```python
from build123d import *

# Parameters (mm, degrees)
SKETCH001_W       = 0.6
SKETCH001_H       = 18.5
PAD001_DEPTH      = 3
PAD002_DEPTH      = 9
PAD002_DEPTH_BACK = 3
FILLET_R          = 1
FILLET001_R       = 2


with BuildPart() as part:
    # Sketch001 → Pad001 (new body)
    with BuildSketch(Plane.YZ):
        Polygon((-13, 10.5), (-13, -10.5), (0, -10.5), (0, -7.5), (-7, -7.5), (-7, 7.5), (0, 7.5), (0, 21.5), (-2.5, 21.5), (-5, 10.5), align=None)
        with Locations((-11, 0)):
            Rectangle(SKETCH001_W, SKETCH001_H, mode=Mode.SUBTRACT)
    extrude(amount=PAD001_DEPTH)

    # Sketch002 (on Face16 of Pad001) → Pad002 (join, two sides)
    with BuildSketch(Plane.YZ.offset(3)) as pad002_sk:
        with BuildLine():
            ThreePointArc((-2.457456, 26.343228), (-2.661032, 23.237253), (0, 21.622499))
            Line((0, 21.622499), (0, 20.622499))
            ThreePointArc((-3.276608, 26.916805), (-3.548043, 22.775505), (0, 20.622499))
            Line((-2.457456, 26.343228), (-3.276608, 26.916805))
        make_face()
    extrude(amount=PAD002_DEPTH)
    extrude(pad002_sk.sketch, amount=-PAD002_DEPTH_BACK)

    # Mirrored: part across XZ


with BuildPart() as part_1:
    add(part.part)
    add(part.part.mirror(Plane.XZ))

    # Fillet
    fillet_edges = [part_1.edges().sort_by_distance(p)[0] for p in [
        (1.5, 13, 10.5),
        (1.5, 13, -10.5),
        (1.5, -13, -10.5),
        (1.5, -13, 10.5),
    ]]
    fillet(fillet_edges, radius=FILLET_R)

    # Fillet001
    fillet001_edges = [part_1.edges().sort_by_distance(p)[0] for p in [
        (1.5, -5, 10.5),
        (1.5, 5, 10.5),
    ]]
    fillet(fillet001_edges, radius=FILLET001_R)


solid = part_1.part
```
Could you check a few things on this model? Use its own coordinates, in mm. A direction names the side the tool comes from. Coordinates: 2 decimals unless noted, no trailing zeros. Write each loop counter-clockwise with the first axis right and the second up, starting at its lowest first coordinate (ties: lowest second). Pieces come first, ordered by that corner, then holes. Notation, with made-up numbers: (64, 32.25) -> (123, 32.25) arc R22 cw to (123, 54.25) -> close; hole circle Ø3 at (-20, -35.5). An arc over 180 degrees is marked (long way). Write item = value, one per line. Start each with the question number.
(1) I need wall thicknesses on line 1 (Y direction, x = 2, z = 6); line 2 (Z direction, x = 1.5, y = 6.75); line 3 (Z direction, x = 2, y = -11.25). Which ranges of each line are inside material? Lowest first, please. Write a range as [from, to].
(2) I want a section at C-C (y = -5.5). Please give me the cut outline in (x, z), plus the area to 3 significant figures.
(3) Which directions (+Z, -Z, +X, -X, +Y, -Y) give clear straight access to the entire face, cutting with the end or side of a thin tool? Please do faces 1 (the face through (1.48, 3.56, 16.84)), 2 (the face through (1, -10.7, 0)), 3 (the face through (1, -9, 10.5)), 4 (the face through (6.084, -2.861, 26.626)).
(4) I want a section at B-B (z = 0.5). Please give me the cut outline in (x, y).
(5) I want a section at D-D (x = 8.5). Please give me the cut outline in (y, z), plus the area to 3 significant figures.
(6) Will these pins go through, and if not, where does the flat tip stop? pin 1 (1.5 mm diameter, centred on y = -4.5, z = 8.5, fed in from -X); pin 2 (6 mm diameter, centred on x = 4.5, y = 8, fed in from +Z); pin 3 (1.5 mm diameter, centred on x = 2, y = -10, fed in from +Z); pin 4 (2 mm diameter, centred on x = 5, y = -4, fed in from -Z).
(7) I want a section at A-A (x = 2.25). Give the number of separate pieces and of enclosed holes in the cut face, plus the area to 3 significant figures.
(8) We'd pull the mould along Z, two halves only. Please class faces 5 (the face through (6.084, 2.861, 26.626)), 6 (the face through (12, 0, 21)), 7 (the face through (1, 11.3, 0)): released by +Z, released by -Z, zero draft, split by the parting line, or undercut.
Result set:
q1.line_1 = [-13, -11.3], [-10.7, -7], [7, 10.7], [11.3, 13]
q1.line_2 = [-10.5, -7.5], [7.5, 10.5]
q1.line_3 = [-10.5, -9.25], [9.25, 10.5]
q2.outline = (0, -10.5) -> (3, -10.5) -> (3, -7.5) -> (0, -7.5) -> close; (0, 7.5) -> (3, 7.5) -> (3, 10.83) -> (0, 10.83) -> close
q2.area = 19.0 mm2
q3.face_1 = +X, -X, +Y
q3.face_2 = +X, -X
q3.face_3 = +Z, +X, -X, -Y
q3.face_4 = +Z, +X, -X
q4.outline = (0, -13) -> (3, -13) -> (3, -11.3) -> (0, -11.3) -> close; (0, -10.7) -> (3, -10.7) -> (3, -7) -> (0, -7) -> close; (0, 7) -> (3, 7) -> (3, 10.7) -> (0, 10.7) -> close; (0, 11.3) -> (3, 11.3) -> (3, 13) -> (0, 13) -> close
q5.outline = (-3.28, 26.92) arc R4 ccw to (0, 20.62) arc R4 ccw to (3.28, 26.92) -> (2.46, 26.34) arc R3 cw (long way) to (-2.46, 26.34) -> close
q5.area = 15.3 mm2
q6.pin_1 = 0
q6.pin_2 = 10.9
q6.pin_3 = 10.5
q6.pin_4 = 21.98
q7.separate_pieces = 1
q7.enclosed_holes = 3
q7.area = 409 mm2
q8.face_5 = released by +Z
q8.face_6 = zero draft
q8.face_7 = undercut
